Verification items for the finished model (mm, model axes). A direction names the side the tool comes from. Give positions to 0.01 mm unless a question says otherwise; leave off trailing zeros. Write each loop counter-clockwise with the first axis right and the second up, starting at its lowest first coordinate (ties: lowest second). Pieces come first, ordered by that corner, then holes. Notation, with made-up numbers: (26, -18.5) - (60, -18.5) arc R20 ccw to (60, -9.5) - close; hole circle Ø3 at (-13, 27.25). An arc over 180 degrees is marked (long way). Put each result on its own line as item: value.
from build123d import *

# Parameters (mm, degrees)
F1_DEPTH = 50
F3_DEPTH = 50
F5_DEPTH = 74.7484416821


with BuildPart() as f1:
    # F0 (on Top) → F1 (new body)
    with BuildSketch(Plane.XY):
        Polygon((36.7763043397, 0), (0, 33.874820134), (-36.7763043397, 0), (0, -33.874820134), align=None)
    extrude(amount=-F1_DEPTH)

    # F2 (on face) → F3 (cut)
    with BuildSketch(Plane(origin=(-16.8803742831, -18.3262310928, 0), x_dir=(0.7355260868, -0.6774964027, 0), z_dir=(-0.6774964027, -0.7355260868, 0))):
        with BuildLine():
            Line((-21.0499312177, -23.8044057041), (-21.0499312177, -50))
            Line((-21.0499312177, -50), (16.9500687823, -50))
            Line((16.9500687823, -50), (16.9500687823, -23.8044057041))
            ThreePointArc((16.9500687823, -23.8044057041), (-2.0499312177, -4.8044057041), (-21.0499312177, -23.8044057041))
        make_face()
    extrude(amount=-F3_DEPTH, mode=Mode.SUBTRACT)

    # F4 (on face) → F5 (cut, through all)
    with BuildSketch(Plane(origin=(16.8803742831, -18.3262310928, 0), x_dir=(0.7355260868, 0.6774964027, 0), z_dir=(0.6774964027, -0.7355260868, 0))):
        with BuildLine():
            Line((-16.9500687823, -22.5290991366), (-16.9500687823, -50))
            Line((-16.9500687823, -50), (21.0499312177, -50))
            Line((21.0499312177, -50), (21.0499312177, -22.5290991366))
            ThreePointArc((21.0499312177, -22.5290991366), (2.0499312177, -3.5290991366), (-16.9500687823, -22.5290991366))
        make_face()
    extrude(amount=-F5_DEPTH, mode=Mode.SUBTRACT)


solid = f1.part
Q1. Section check B-B, the plane z = -21. Record the cut outline in (x, y), plus the area to 3 significant figures.
Answers follow:
outline: (-36.78, 0) - (-32.21, -4.21) - (-25.65, 2.92) - (-29.3, 6.88) - close; (-4.57, -29.67) - (0, -33.87) - (4.46, -29.77) - (-0.1, -24.82) - close; (-1.44, 32.55) - (0.1, 30.87) - (1.55, 32.45) - (0, 33.87) - close; (25.65, 3.13) - (32.32, -4.11) - (36.78, 0) - (29.19, 6.98) - close
area: 160 mm2
Q2. Section check A-A, the plane z = -38. Record the cut outline in (x, y), plus the area to 3 significant figures.
Answers follow:
outline: (-36.78, 0) - (-32.36, -4.06) - (-25.83, 3.03) - (-29.35, 6.84) - close; (-4.41, -29.81) - (0, -33.87) - (4.41, -29.81) - (0, -25.02) - close; (-1.4, 32.59) - (0, 31.07) - (1.4, 32.59) - (0, 33.87) - close; (25.83, 3.03) - (32.36, -4.06) - (36.78, 0) - (29.35, 6.84) - close
area: 153 mm2
Q3. Scan lines: line 1 along Z through (x, y) = (6, -13.5); line 2 along X through (y, z) = (-5, -14.5); line 3 along Z through (x, y) = (-11, -22.5). Record each from-to range of solid material in increasing order.
Answers follow:
line 1: z = -4.78 to 0
line 2: x = -31.35 to -29.92, 30.8 to 31.35
line 3: z = -7.18 to 0
Q4. Set-up check for faces 4 (the face through (2.22, -27.43, -36.07)), 5 (the face through (-2.24, -27.45, -37.09)), 6 (the face through (-29.143, -0.569, -36.719)): record each of +Z, -Z, +X, -X, +Y, -Y from which the full face is reachable in a straight line by a thin tool's end or side.
Answers follow:
face 4: -Z, +X
face 5: -Z, -X
face 6: -Z, -Y
Q5. Go/stop test with flat-tipped pins: pin 1 Ø4 at (y, z) = (-4.5, -7) entering from -X; pin 2 Ø3 at (x, z) = (-24.5, -32.5) entering from -Y; pin 3 Ø4 at (x, y) = (10, 4.5) entering from -Z; pin 4 Ø10 at (x, z) = (-11, -40) entering from -Y. Record where each tip stops, or that it passes through.
Answers follow:
pin 1: stops at x = -34.06
pin 2: stops at y = 2.84
pin 3: stops at z = -6.39
pin 4: passes through
Q6. Release check for a two-part mould opening along Y. For faces 1 (the face through (-27.55, 4.89, -36.07)), 2 (the face through (-31, 1, -50)), 3 (the face through (11.43, 14.82, -4.81)) record: released by +Y, released by -Y, zero draft, split by the parting line, or undercut.
Answers follow:
face 1: released by +Y
face 2: zero draft
face 3: undercut
